from build123d import *

# Parameters (mm, degrees)
SKETCH1_W           = 28
SKETCH1_H           = 16.1
BOSS_EXTRUDE1_DEPTH = 30
SKETCH2_W           = 10
SKETCH2_H           = 2.5
CUT_EXTRUDE1_DEPTH  = 5
SKETCH3_W           = 10
SKETCH3_H           = 4
CUT_EXTRUDE2_DEPTH  = 8
SKETCH4_W           = 10
SKETCH4_H           = 3.2
CUT_EXTRUDE3_DEPTH  = 8
SKETCH5_W           = 11
SKETCH5_H           = 4
CUT_EXTRUDE4_DEPTH  = 8
SKETCH6_W           = 20
SKETCH6_H           = 2
BOSS_EXTRUDE2_DEPTH = 5
CHAMFER1_SIZE       = 4
SKETCH7_W           = 20
SKETCH7_H           = 2
BOSS_EXTRUDE3_DEPTH = 5
CHAMFER2_SIZE       = 4
SKETCH9_W           = 25.8
SKETCH9_H           = 19
CUT_EXTRUDE6_DEPTH  = 10
SKETCH13_R          = 4.1
CUT_EXTRUDE10_DEPTH = 27.2
SKETCH14_R          = 4.1
CUT_EXTRUDE11_DEPTH = 27.2
SKETCH15_W          = 8.2
SKETCH15_H          = 4
CUT_EXTRUDE12_DEPTH = 27.2
SKETCH16_W          = 0.59230819
SKETCH16_H          = 0.8
SKETCH16_W_2        = 1.617695922
CUT_EXTRUDE13_DEPTH = 4
SKETCH17_W          = 1.5
SKETCH17_H          = 4
BOSS_EXTRUDE4_DEPTH = 16.1
FILLET1_R           = 0.5
SKETCH18_R          = 3.5
CUT_EXTRUDE14_DEPTH = 6.1
SKETCH19_W          = 8
SKETCH19_H          = 1
CUT_EXTRUDE15_DEPTH = 10
SKETCH20_W          = 20.5
SKETCH20_H          = 10.6
CUT_EXTRUDE16_DEPTH = 1.5
SKETCH21_W          = 5.7
SKETCH21_H          = 8
CUT_EXTRUDE17_DEPTH = 1.5
SKETCH22_W          = 8
SKETCH22_H          = 2.5
CUT_EXTRUDE18_DEPTH = 1.5
SKETCH23_R          = 1.15
CUT_EXTRUDE19_DEPTH = 75.620049118
SKETCH24_W          = 8.2
SKETCH24_H          = 0.8
CUT_EXTRUDE20_DEPTH = 2.1
CUT_EXTRUDE21_REACH = 75.421
SKETCH25_W          = 7.929527271
SKETCH25_H          = 0.8
CUT_EXTRUDE22_START = -5
SKETCH26_W          = 4
SKETCH26_H          = 6
CUT_EXTRUDE22_DEPTH = 5
CUT_EXTRUDE23_START = -5
SKETCH27_W          = 4
SKETCH27_H          = 6
CUT_EXTRUDE23_DEPTH = 5
SKETCH28_R          = 1.15
CUT_EXTRUDE24_DEPTH = 3.2
CUT_EXTRUDE25_REACH = 75.764
SKETCH29_W          = 15.5
SKETCH29_H          = 10.6


with BuildPart() as part:
    # Sketch1 → Boss-Extrude1 (new body)
    with BuildSketch(Plane(origin=(0, 0, 0), x_dir=(0, 0, -1), z_dir=(1, 0, 0))):
        with Locations((-46.701535197, -0.990821865)):
            Rectangle(SKETCH1_W, SKETCH1_H)
    extrude(amount=BOSS_EXTRUDE1_DEPTH)

    # Sketch2 → Cut-Extrude1 (cut)
    with BuildSketch(Plane.XY.offset(60.701535197)):
        with Locations((25, 5.809178135)):
            Rectangle(SKETCH2_W, SKETCH2_H)
    extrude(amount=-CUT_EXTRUDE1_DEPTH, mode=Mode.SUBTRACT)

    # Sketch3 → Cut-Extrude2 (cut)
    with BuildSketch(Plane.XY.offset(60.701535197)):
        with Locations((5, 5.059178135)):
            Rectangle(SKETCH3_W, SKETCH3_H)
    extrude(amount=-CUT_EXTRUDE2_DEPTH, mode=Mode.SUBTRACT)

    # Sketch4 → Cut-Extrude3 (cut)
    with BuildSketch(Plane(origin=(0, 0, 32.701535197), x_dir=(-1, 0, 0), z_dir=(0, 0, -1))):
        with Locations((-6, 5.459178135)):
            Rectangle(SKETCH4_W, SKETCH4_H)
    extrude(amount=-CUT_EXTRUDE3_DEPTH, mode=Mode.SUBTRACT)

    # Sketch5 → Cut-Extrude4 (cut)
    with BuildSketch(Plane(origin=(0, 0, 32.701535197), x_dir=(-1, 0, 0), z_dir=(0, 0, -1))):
        with Locations((-24.5, 5.059178135)):
            Rectangle(SKETCH5_W, SKETCH5_H)
    extrude(amount=-CUT_EXTRUDE4_DEPTH, mode=Mode.SUBTRACT)

    # Sketch6 → Boss-Extrude2 (add)
    with BuildSketch(Plane(origin=(0, 0, 32.701535197), x_dir=(-1, 0, 0), z_dir=(0, 0, -1))):
        with Locations((-20, -4.040821865)):
            Rectangle(SKETCH6_W, SKETCH6_H)
    extrude(amount=BOSS_EXTRUDE2_DEPTH)

    # Chamfer1
    chamfer1_edges = [part.edges().sort_by_distance(p)[0] for p in [
        (20, -3.040821865, 32.701535197),
    ]]
    chamfer(chamfer1_edges, length=CHAMFER1_SIZE)

    # Sketch7 → Boss-Extrude3 (add)
    with BuildSketch(Plane.XY.offset(60.701535197)):
        with Locations((10, -4.040821865)):
            Rectangle(SKETCH7_W, SKETCH7_H)
    extrude(amount=BOSS_EXTRUDE3_DEPTH)

    # Chamfer2
    chamfer2_edges = [part.edges().sort_by_distance(p)[0] for p in [
        (10, -3.040821865, 60.701535197),
    ]]
    chamfer(chamfer2_edges, length=CHAMFER2_SIZE)

    # Sketch9 → Cut-Extrude6 (cut)
    with BuildSketch(Plane(origin=(0, 7.059178135, 0), x_dir=(1, 0, 0), z_dir=(0, 1, 0))):
        with Locations((13.9, -46.701535197)):
            Rectangle(SKETCH9_W, SKETCH9_H)
    extrude(amount=-CUT_EXTRUDE6_DEPTH, mode=Mode.SUBTRACT)

    # Sketch13 → Cut-Extrude10 (cut)
    with BuildSketch(Plane.XY.offset(60.701535197)):
        with Locations((21.482304078, -9.040821865)):
            Circle(SKETCH13_R)
    extrude(amount=-CUT_EXTRUDE10_DEPTH, mode=Mode.SUBTRACT)

    # Sketch14 → Cut-Extrude11 (cut)
    with BuildSketch(Plane(origin=(0, 0, 32.701535197), x_dir=(-1, 0, 0), z_dir=(0, 0, -1))):
        with Locations((-6.49230819, -9.040821865)):
            Circle(SKETCH14_R)
    extrude(amount=-CUT_EXTRUDE11_DEPTH, mode=Mode.SUBTRACT)

    # Sketch15 → Cut-Extrude12 (cut)
    with BuildSketch(Plane.XZ.offset(9.040821865)):
        with Locations((6.49230819, 57.901535197)):
            Rectangle(SKETCH15_W, SKETCH15_H)
        with Locations((21.482304078, 35.501535197)):
            Rectangle(SKETCH15_W, SKETCH15_H)
    extrude(amount=-CUT_EXTRUDE12_DEPTH, mode=Mode.SUBTRACT)

    # Sketch16 → Cut-Extrude13 (cut)
    with BuildSketch(Plane(origin=(0, 7.059178135, 0), x_dir=(1, 0, 0), z_dir=(0, 1, 0))):
        with Locations((10.296154095, -60.301535197)):
            Rectangle(SKETCH16_W, SKETCH16_H)
        with Locations((18.191152039, -33.101535197)):
            Rectangle(SKETCH16_W_2, SKETCH16_H)
    extrude(amount=-CUT_EXTRUDE13_DEPTH, mode=Mode.SUBTRACT)

    # Sketch17 → Boss-Extrude4 (add)
    with BuildSketch(Plane.XZ.offset(9.040821865)):
        with Locations((30.75, 46.701535197)):
            Rectangle(SKETCH17_W, SKETCH17_H)
    extrude(amount=-BOSS_EXTRUDE4_DEPTH)

    # Fillet1
    fillet1_edges = [part.edges().sort_by_distance(p)[0] for p in [
        (30, -0.990821865, 44.701535197),
        (30, -0.990821865, 48.701535197),
        (31.5, -0.990821865, 48.701535197),
        (31.5, -0.990821865, 44.701535197),
    ]]
    fillet(fillet1_edges, radius=FILLET1_R)

    # Sketch18 → Cut-Extrude14 (cut)
    with BuildSketch(Plane.XZ.offset(9.040821865)):
        with Locations(Location((13.985, 46.701535197, 0), (0, 0, 194.224464848))):
            Circle(SKETCH18_R)
    extrude(amount=-CUT_EXTRUDE14_DEPTH, mode=Mode.SUBTRACT)

    # Sketch19 → Cut-Extrude15 (cut)
    with BuildSketch(Plane(origin=(31.5, 0, 0), x_dir=(0, 0, -1), z_dir=(1, 0, 0))):
        with Locations((-46.701535197, -2.440821865)):
            Rectangle(SKETCH19_W, SKETCH19_H)
    extrude(amount=-CUT_EXTRUDE15_DEPTH, mode=Mode.SUBTRACT)

    # Sketch20 → Cut-Extrude16 (cut)
    with BuildSketch(Plane(origin=(0, -2.940821865, 0), x_dir=(1, 0, 0), z_dir=(0, 1, 0))):
        with Locations((14.05, -46.701535197)):
            Rectangle(SKETCH20_W, SKETCH20_H)
    extrude(amount=-CUT_EXTRUDE16_DEPTH, mode=Mode.SUBTRACT)

    # Sketch21 → Cut-Extrude17 (cut)
    with BuildSketch(Plane(origin=(0, -2.940821865, 0), x_dir=(1, 0, 0), z_dir=(0, 1, 0))):
        with Locations((27.15, -46.701535197)):
            Rectangle(SKETCH21_W, SKETCH21_H)
    extrude(amount=-CUT_EXTRUDE17_DEPTH, mode=Mode.SUBTRACT)

    # Sketch22 → Cut-Extrude18 (cut)
    with BuildSketch(Plane(origin=(31.5, 0, 0), x_dir=(0, 0, -1), z_dir=(1, 0, 0))):
        with Locations((-46.701535197, -3.190821865)):
            Rectangle(SKETCH22_W, SKETCH22_H)
    extrude(amount=-CUT_EXTRUDE18_DEPTH, mode=Mode.SUBTRACT)

    # Sketch23 → Cut-Extrude19 (cut, through all)
    with BuildSketch(Plane(origin=(0, 7.059178135, 0), x_dir=(1, 0, 0), z_dir=(0, 1, 0))):
        with Locations(Location((29, -46.701535197, 0), (0, 0, 270))):
            Circle(SKETCH23_R)
        with Locations(Location((14, -34.951535197, 0), (0, 0, 270))):
            Circle(SKETCH23_R)
        with Locations(Location((14, -58.451535197, 0), (0, 0, 270))):
            Circle(SKETCH23_R)
    extrude(amount=-CUT_EXTRUDE19_DEPTH, mode=Mode.SUBTRACT)

    # Sketch24 → Cut-Extrude20 (cut)
    with BuildSketch(Plane(origin=(0, 3.059178135, 0), x_dir=(1, 0, 0), z_dir=(0, 1, 0))):
        with Locations((21.482304078, -33.101535197)):
            Rectangle(SKETCH24_W, SKETCH24_H)
        with Locations((6.49230819, -60.301535197)):
            Rectangle(SKETCH24_W, SKETCH24_H)
    extrude(amount=-CUT_EXTRUDE20_DEPTH, mode=Mode.SUBTRACT)

    # Cut-Extrude21: up to this face of the body (flat: up to its plane)
    cut_extrude21_end = Plane(part.part.faces().sort_by_distance((30, -1.445232759, 54.822020691))[0])
    # Sketch25 → Cut-Extrude21 (cut, up to the picked face)
    with BuildSketch(Plane(origin=(31.5, 0, 0), x_dir=(0, 0, -1), z_dir=(1, 0, 0)), mode=Mode.PRIVATE) as cut_extrude21_sk1:
        with Locations((-46.553400254, 6.659178135)):
            Rectangle(SKETCH25_W, SKETCH25_H)
    cut_extrude21_tool1 = split(extrude(cut_extrude21_sk1.sketch, amount=-CUT_EXTRUDE21_REACH, mode=Mode.PRIVATE), bisect_by=cut_extrude21_end, keep=Keep.BOTH, mode=Mode.PRIVATE)
    add(cut_extrude21_tool1.solids().sort_by(Axis((31.5, 6.659178, 46.5534), (-1, 0, 0)))[0], mode=Mode.SUBTRACT)

    # Sketch26 → Cut-Extrude22 (cut)
    with BuildSketch(Plane.XY.offset(65.701535197).offset(CUT_EXTRUDE22_START)):
        with Locations((10, -2.040821865)):
            Rectangle(SKETCH26_W, SKETCH26_H)
    extrude(amount=CUT_EXTRUDE22_DEPTH, mode=Mode.SUBTRACT)

    # Sketch27 → Cut-Extrude23 (cut)
    with BuildSketch(Plane(origin=(0, 0, 27.701535197), x_dir=(-1, 0, 0), z_dir=(0, 0, -1)).offset(CUT_EXTRUDE23_START)):
        with Locations((-20, -2.040821865)):
            Rectangle(SKETCH27_W, SKETCH27_H)
    extrude(amount=CUT_EXTRUDE23_DEPTH, mode=Mode.SUBTRACT)

    # Sketch28 → Cut-Extrude24 (cut)
    with BuildSketch(Plane(origin=(30, 0, 0), x_dir=(0, 0, -1), z_dir=(1, 0, 0))):
        with Locations((-55.201535197, -1.540821865)):
            Circle(SKETCH28_R)
        with Locations((-38.201535197, -1.540821865)):
            Circle(SKETCH28_R)
    extrude(amount=-CUT_EXTRUDE24_DEPTH, mode=Mode.SUBTRACT)

    # Cut-Extrude25: up to this face of the body (flat: up to its plane)
    cut_extrude25_end = Plane(part.part.faces().sort_by_distance((10.921875254, -9.040821865, 51.731547487))[0])
    # Sketch29 → Cut-Extrude25 (cut, up to the picked face)
    with BuildSketch(Plane(origin=(0, -4.440821865, 0), x_dir=(1, 0, 0), z_dir=(0, 1, 0)), mode=Mode.PRIVATE) as cut_extrude25_sk1:
        with Locations((14.05, -46.701535197)):
            Rectangle(SKETCH29_W, SKETCH29_H)
    cut_extrude25_tool1 = split(extrude(cut_extrude25_sk1.sketch, amount=-CUT_EXTRUDE25_REACH, mode=Mode.PRIVATE), bisect_by=cut_extrude25_end, keep=Keep.BOTH, mode=Mode.PRIVATE)
    add(cut_extrude25_tool1.solids().sort_by(Axis((14.05, -4.440822, 46.701535), (0, -1, 0)))[0], mode=Mode.SUBTRACT)


solid = part.part
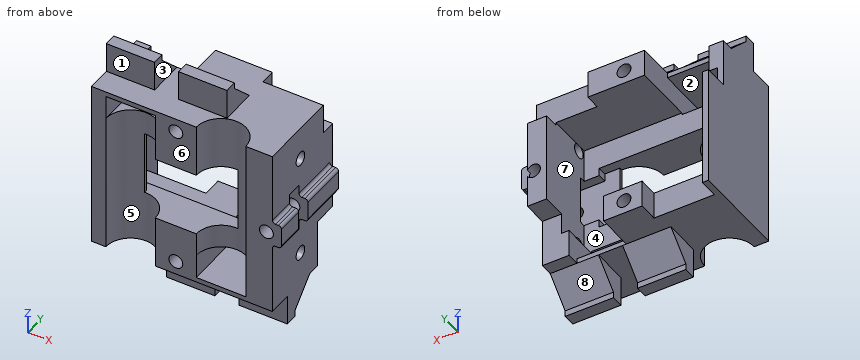
Work out the finished part from the listing and answer in its coordinate system (mm). Face numbers are marked on the shaded views. A direction names the side the tool comes from. Coordinates: 2 decimals unless noted, no trailing zeros. Write each loop counter-clockwise with the first axis right and the second up, starting at its lowest first coordinate (ties: lowest second). Pieces come first, ordered by that corner, then holes. Notation, with made-up numbers: M -4.5,27 L 2.5,27 A17 cw 2.5,38 Z; hole C 77.25,48.5 d5. An arc over 180 degrees is marked long. Answer as CSV lines item,"result". Start each with the question number.
Item 1: Section B-B on x = 29 is taken. Write down the section's boundary in (y, z).
Item 2: Section C-C on x = 7.5 is taken. Write down the section's boundary in (y, z), and give its area (3 significant figures).
Item 3: Consider L1, parallel to X at y = 2.5, z = 44; L2, parallel to Z at x = 29, y = 3.25; L3, parallel to X at y = -6.5, z = 41. Determine where each line is inside the solid, lowest interval first.
Item 4: Section A-A on x = 14 is taken. Give the number of separate pieces and of enclosed holes in the cut face, and give its area (3 significant figures).
Item 5: A tool of negligible diameter and unlimited length cuts with its end or side. For the marked faces 1, 2, 3, 4 and 5, from which of +Z, -Z, +X, -X, +Y, -Y can it reach the whole face along a straight path? Write none if from no direction.
Item 6: Section D-D on z = 59 is taken. Write down the section's boundary in (x, y), and give its area (3 significant figures).
Item 7: Flat-ended cylindrical pins translate along their axes: P1, Ø3.5, axis at x = 6, z = 34, coming from the +Y side; P2, Ø1.5, axis at y = -1.5, z = 57, coming from the +X side; P3, Ø3, axis at x = 7.5, y = -7, coming from the +Z side; P4, Ø1.8, axis at x = 14, z = 34.95, coming from the -Y side. Find the tip coordinate at first contact, or state that the pin passes through.
Item 8: Determine the mould class of the marked faces 6, 7 and 8 for opening direction Z: released by +Z, released by -Z, zero draft, split by the parting line, or undercut.
Checks:
1,outline,"M -9.04,32.7 L -5.04,32.7 L -5.04,27.7 L -3.04,27.7 L -3.04,28.7 L 0.96,32.7 L 3.06,32.7 L 3.06,40.7 L 7.06,40.7 L 7.06,45.55 L -1.94,45.55 L -1.94,42.7 L -4.44,42.7 L -4.44,45.55 L -9.04,45.55 Z; M -9.04,47.85 L -4.44,47.85 L -4.44,50.7 L -1.94,50.7 L -1.94,47.85 L 7.06,47.85 L 7.06,55.7 L 4.56,55.7 L 4.56,60.7 L -9.04,60.7 Z; hole C -1.54,38.2 d2.3; hole C -1.54,55.2 d2.3"
2,outline,"M -9.04,59.9 L 0.96,59.9 L 0.96,60.7 L -3.04,64.7 L -3.04,65.7 L -5.04,65.7 L -5.04,60.7 L -9.04,60.7 Z; M -5.07,32.7 L 3.86,32.7 L 3.86,37.2 L -2.94,37.2 L -2.94,41.4 L -5.07,41.4 Z; M -5.07,52 L -2.94,52 L -2.94,55.9 L -5.07,55.9 Z"
2,area,"83.4 mm²"
3,L1,"x = 0 to 1, 26.8 to 30"
3,L2,"z = 40.7 to 45.55, 47.85 to 60.7"
3,L3,"x = 0 to 3.27, 9.71 to 18.26, 24.7 to 30"
4,separate pieces,"4"
4,enclosed holes,"0"
4,area,"158 mm²"
5,face 1,"+Z, +X, -X, -Y"
5,face 2,"+Y, -Y"
5,face 3,"+Z, +Y, -Y"
5,face 4,"+Y"
5,face 5,"-Z, -Y"
6,outline,"M 0,-9.04 L 2.39,-9.04 L 2.39,3.06 L 0,3.06 Z; M 10.59,-9.04 L 12.99,-9.04 L 12.99,7.06 L 10.59,7.06 Z; M 15.01,-9.04 L 17.38,-9.04 A4.1 cw 25.58,-9.04 L 30,-9.04 L 30,4.56 L 20,4.56 L 20,7.06 L 15.01,7.06 Z"
6,area,"257 mm²"
7,P1,"stops at y = 3.86"
7,P2,"stops at x = 30"
7,P3,"stops at z = 60.7"
7,P4,"passes through"
8,face 6,"zero draft"
8,face 7,"undercut"
8,face 8,"released by -Z"
